from build123d import *

# Parameters (mm, degrees)
BOSS_EXTRUDE1_DEPTH = 30
SKETCH4_W           = 4
SKETCH4_H           = 19
CUT_EXTRUDE3_DEPTH  = 8.5
SKETCH7_R           = 16.05
CUT_EXTRUDE4_DEPTH  = 27
SKETCH6_R           = 9
CUT_EXTRUDE5_DEPTH  = 4
FILLET3_R           = 3
FILLET4_R           = 3
SKETCH8_R           = 1.85
CUT_EXTRUDE6_DEPTH  = 4
SKETCH9_R           = 3
CUT_EXTRUDE7_DEPTH  = 37


with BuildPart() as part:
    # Sketch1 → Boss-Extrude1 (new body)
    with BuildSketch(Plane(origin=(0, 0, 0), x_dir=(1, 0, 0), z_dir=(0, 1, 0))):
        with BuildLine():
            Line((-30, -2), (-30, 2))
            Line((-30, 2), (-17.838231415, 2))
            ThreePointArc((-17.838231415, 2), (0, 17.95), (17.838231415, 2))
            Line((17.838231415, 2), (30, 2))
            Line((30, 2), (30, -2))
            Line((30, -2), (17.838231415, -2))
            ThreePointArc((17.838231415, -2), (0, -17.95), (-17.838231415, -2))
            Line((-17.838231415, -2), (-30, -2))
        make_face()
    extrude(amount=BOSS_EXTRUDE1_DEPTH)

    # Sketch4 → Cut-Extrude3 (cut)
    with BuildSketch(Plane.ZY.offset(30)):
        with Locations((0, 9.5)):
            Rectangle(SKETCH4_W, SKETCH4_H)
    cut_extrude3 = extrude(amount=-CUT_EXTRUDE3_DEPTH, mode=Mode.SUBTRACT)

    # Mirror1: Cut-Extrude3 across plane
    add(cut_extrude3.mirror(Plane(origin=(0, 0, 0), x_dir=(0, 0, 1), z_dir=(1, 0, 0))), mode=Mode.SUBTRACT)

    # Sketch7 → Cut-Extrude4 (cut)
    with BuildSketch(Plane(origin=(0, 30, 0), x_dir=(1, 0, 0), z_dir=(0, 1, 0))):
        with Locations(Location((0, 0, 0), (0, 0, 270))):
            Circle(SKETCH7_R)
    extrude(amount=-CUT_EXTRUDE4_DEPTH, mode=Mode.SUBTRACT)

    # Sketch6 → Cut-Extrude5 (cut)
    with BuildSketch(Plane.XZ):
        with Locations(Location((0, 0, 0), (0, 0, 270))):
            Circle(SKETCH6_R)
    extrude(amount=-CUT_EXTRUDE5_DEPTH, mode=Mode.SUBTRACT)

    # Fillet3
    fillet3_edges = [part.edges().sort_by_distance(p)[0] for p in [
        (-17.838231415, 15, 2),
        (-17.838231415, 15, -2),
        (17.838231415, 15, -2),
        (17.838231415, 15, 2),
    ]]
    fillet(fillet3_edges, radius=FILLET3_R)

    # Fillet4
    fillet4_edges = [part.edges().sort_by_distance(p)[0] for p in [
        (-21.5, 19, 0),
        (21.5, 19, 0),
    ]]
    fillet(fillet4_edges, radius=FILLET4_R)

    # Sketch8 → Cut-Extrude6 (cut)
    with BuildSketch(Plane(origin=(0, 0, -2), x_dir=(-1, 0, 0), z_dir=(0, 0, -1))):
        with Locations((-25.17, 24.5)):
            Circle(SKETCH8_R)
        with Locations(Location((25.17, 24.5, 0), (0, 0, 180))):
            Circle(SKETCH8_R)
    extrude(amount=-CUT_EXTRUDE6_DEPTH, mode=Mode.SUBTRACT)

    # Sketch9 → Cut-Extrude7 (cut)
    with BuildSketch(Plane(origin=(0, 0, -17.95), x_dir=(-1, 0, 0), z_dir=(0, 0, -1))):
        with Locations((0, 18)):
            Circle(SKETCH9_R)
    extrude(amount=-CUT_EXTRUDE7_DEPTH, mode=Mode.SUBTRACT)


solid = part.part
The model under review builds one solid part; all positions refer to its coordinate system, in mm. A direction names the side the tool comes from. Round coordinates to 2 decimals unless told otherwise and drop trailing zeros. Loops run counter-clockwise (first coordinate to the right, second up) from the corner with the lowest first, then second, coordinate; pieces in that order, holes last. Notation, with made-up numbers: M 33.25,48.25 L 82.25,48.25 A23 cw 82.25,84.25 Z; hole C 37,27.5 d4. An arc over 180 degrees is marked long. Answer as CSV lines item,"result".
1. We need section A-A (z = 0). Give the boundary of the cut face in (x, y).
Outcome:
outline,"M -30,19 L -24.5,19 A3 cw -21.5,16 L -21.5,0 L -9,0 L -9,3 L -16.05,3 L -16.05,30 L -30,30 Z; M 9,0 L 21.5,0 L 21.5,16 A3 cw 24.5,19 L 30,19 L 30,30 L 16.05,30 L 16.05,3 L 9,3 Z; hole C -25.17,24.5 d3.7; hole C 25.17,24.5 d3.7"
2. To check wall thickness, follow L1, parallel to Y at x = 25, z = -1; L2, parallel to Y at x = 0, z = -16.6; L3, parallel to X at y = 12.5, z = 0. State the ranges of each line that lie inside material, in increasing order. Write a range as [from, to].
Outcome:
L1,"y = [19, 22.66], [26.34, 30]"
L2,"y = [0, 15], [21, 30]"
L3,"x = [-21.5, -16.05], [16.05, 21.5]"
3. Draft analysis for pull direction Z (two halves, no side actions). For faces 1 (the face through (-6.147, 16.689, 14.826)), 2 (the face through (18.47, 15.21, -2.66)), 3 (the face through (0.334, 14.79, 17.947)), state which applies: pulls with the +Z half, pulls with the -Z half, needs draft (parallel to the pull), parting line crosses it, or undercut.
Outcome:
face 1,"undercut"
face 2,"pulls with the -Z half"
face 3,"pulls with the +Z half"
4. We need section B-B (y = 24.5). Give the boundary of the cut face in (x, z).
Outcome:
outline,"M -30,-2 L -27.02,-2 L -27.02,2 L -30,2 Z; M -23.32,-2 L -20.34,-2 A3 cw -17.43,-4.28 A17.95 ccw 17.43,-4.28 A3 cw 20.34,-2 L 23.32,-2 L 23.32,2 L 20.34,2 A3 cw 17.43,4.28 A17.95 ccw -17.43,4.28 A3 cw -20.34,2 L -23.32,2 Z; M 27.02,-2 L 30,-2 L 30,2 L 27.02,2 Z; hole C 0,0 d32.1"
5. We need section C-C (x = 25.17). Give the boundary of the cut face in (y, z).
Outcome:
outline,"M 19,-2 L 22.65,-2 L 22.65,2 L 19,2 Z; M 26.35,-2 L 30,-2 L 30,2 L 26.35,2 Z"
6. We need section D-D (x = 0). Give the boundary of the cut face in (y, z).
Outcome:
outline,"M 0,-17.95 L 15,-17.95 L 15,-16.05 L 3,-16.05 L 3,-9 L 0,-9 Z; M 0,9 L 3,9 L 3,16.05 L 15,16.05 L 15,17.95 L 0,17.95 Z; M 21,-17.95 L 30,-17.95 L 30,-16.05 L 21,-16.05 Z; M 21,16.05 L 30,16.05 L 30,17.95 L 21,17.95 Z"
7. Insertion check: pin 1 Ø5 at (y, z) = (5, 13.5) entering from -X; pin 2 Ø5 at (x, y) = (0, 18) entering from -Z; pin 3 Ø10.5 at (x, y) = (25.5, 9.5) entering from +Z; pin 4 Ø10.5 at (x, y) = (-25.5, 18) entering from -Z. Each pin has a flat end and moves straight along its axis. Give the tip position at first contact, or say it passes through.
Outcome:
pin 1,"stops at x = -14.18"
pin 2,"passes through"
pin 3,"stops at z = 2"
pin 4,"stops at z = -2"
8. For faces 4 (the face through (-24, 21, 2)), 5 (the face through (-27, 19, 0)), 6 (the face through (27, 19, 0)), 7 (the face through (24, 21, 2)), 8 (the face through (-7, 3, 7)), list the 3-axis set-ups (+Z, -Z, +X, -X, +Y, -Y) from which the entire face can be reached by the end or side of a thin tool; tool diameter is ignored.
Outcome:
face 4,"+Z, -X, +Y, -Y"
face 5,"+Z, -Z, -X, -Y"
face 6,"+Z, -Z, +X, -Y"
face 7,"+Z, +X, +Y, -Y"
face 8,"+Y"
